Autodesk Inventor part; units mm, degrees
ref_plane "YZ Plane" through (0, 0, 0) normal (1, 0, 0) x (0, 1, 0)
ref_plane "XZ Plane" through (0, 0, 0) normal (0, 1, 0) x (-1, 0, 0)
ref_plane "XY Plane" through (0, 0, 0) normal (0, 0, 1) x (1, 0, 0)
sketch "Sketch1" plane through (0, 0, 0) normal (0, 0, 1) x (1, 0, 0)
  line L0 (0, -91.8925) -> (0, 152.1979) construction
  line L1 (3.18, 0) -> (7.58, 0)
  line L2 (7.58, 0) -> (7.58, 20)
  line L3 (7.58, 20) -> (3.18, 20)
  line L4 (3.18, 0) -> (3.18, 20)
  point P0 (0, 0)
  dimension "d1" = 3.18
  dimension "d2" = 20
  dimension "d17" = 4.4
  dimension "d18" = 7.58
revolve "Revolution1" add sketch "Sketch1" angle 360 about axis through (0, -91.8925, 0) along (0, 1, 0)
sketch "Sketch2" plane through (0, 0, 0) normal (0, 0, 1) x (1, 0, 0)
  line L0 (3.18, 0) -> (3.18, 20)
  line L1 (-7.58, 20) -> (7.58, 20) construction
  line L2 (7.58, 20) -> (42.58, 20) construction
  line L3 (7.58, 20) -> (7.58, 0)
  line L4 (38.7358, 38.6122) -> (39.7358, 38.6122)
  line L5 (38.7358, 38.6122) -> (33.7358, 38.6122)
  line L6 (39.7358, 38.6122) -> (39.7358, 43.6122)
  line L7 (33.7358, 38.6122) -> (33.7358, 43.6122)
  line L8 (39.7358, 43.6122) -> (41.7358, 43.6122)
  line L9 (41.7358, 43.6122) -> (41.7358, 36.6122)
  line L10 (41.7358, 36.6122) -> (7.58, 11.215)
  line L11 (33.7358, 43.6122) -> (31.7358, 43.6122)
  line L12 (3.18, 20) -> (7.58, 20)
  line L13 (7.58, 11.215) -> (7.58, 20)
  line L14 (0, 30.8602) -> (0, -63.1044)
  line L15 (31.7358, 43.6122) -> (31.7358, 40.4576)
  line L16 (31.7358, 40.4576) -> (3.18, 20)
  point P0 (0, 0)
  dimension "d6" = 35
  dimension "d7" = 1
  dimension "d8" = 5
  dimension "d9" = 5
  dimension "d10" = 5
  dimension "d11" = 2
  dimension "d12" = 7
  dimension "d13" = 2
revolve "Revolution2" add sketch "Sketch2" angle 360 about axis through (0, 30.8602, 0) along (0, -1, 0)
fillet "Fillet1" radius 2 1 edges at (-3.18, 20, 0)
fillet "Fillet2" radius 0.5 4 edges at (-31.7358, 43.6122, 0) (-33.7358, 43.6122, 0) (-39.7358, 43.6122, 0) (-41.7358, 43.6122, 0)
properties part number "Drain Funnel v0.6.2"
Part model, mm, in its own coordinate system. A direction names the side the tool comes from. Coordinates: 2 decimals unless noted, no trailing zeros. Order: outer loops, then holes, each group sorted by start corner. A loop starts at its lowest first (then second) coordinate and runs counter-clockwise, first axis right, second up. Notation, with made-up numbers: (-1.5, 57.25) -> (5.5, 57.25) arc R24 cw to (5.5, 73.25) -> close; hole circle Ø9 at (33.25, 55). An arc over 180 degrees is marked (long way). Put each result on its own line as item: value. Start each with the question number.
(1) Probe line 1 along Z through (x, y) = (0, 42); line 2 along X through (y, z) = (39.5, 14); line 3 along X through (y, z) = (41, 28). List the from-to ranges inside material, lowest first. Write a range as [from, to].
(2) Which spindle directions (+Z, -Z, +X, -X, +Y, -Y) get a long thin tool onto all of the face, cutting with end or side? Do faces 1 (the face through (7.23, 5.69, -2.28)), 2 (the face through (-33.12, 39.817, -25.396)), 3 (the face through (-26.77, 40.89, 20.53)). Say none if no direction does.
(3) Mould opens along X. For faces 4 (the face through (-18, 38.612, -29)), 5 (the face through (-5, 43.612, 32)), 6 (the face through (9.268, 12.804, -2.919)) say: pulls with the +X half, pulls with the -X half, needs draft (parallel to the pull), parting line crosses it, or undercut.
(4) Band-saw the part on A-A (y = 10). Give the cut face in (x, z), then the cut area to 3 significant figures.
(5) Pin check, flat tips, straight feed: pin 1 Ø8 at (x, y) = (12.5, 25.5) entering from +Z; pin 2 Ø4 at (x, z) = (29, 3) entering from -Y; pin 3 Ø2 at (x, z) = (-33, -14.5) entering from -Y; pin 4 Ø5.5 at (x, z) = (0, 0) entering from -Y (3 decimals). Stop position of each tip, or through.
(6) Band-saw the part on B-B (y = 34.5). Give the cut face in (x, z).
Determined:
1. line 1: z = [-41.74, -39.74], [-33.74, -31.74], [31.74, 33.74], [39.74, 41.74]
1. line 2: x = [-39.32, -37.19], [-30.69, -26.98], [26.98, 30.69], [37.19, 39.32]
1. line 3: x = [-30.95, -28.19], [-18.82, -14.94], [14.94, 18.82], [28.19, 30.95]
2. face 1: -Y
2. face 2: +Y, -Y
2. face 3: +Y
3. face 4: undercut
3. face 5: needs draft
3. face 6: parting line crosses it
4. outline: circle Ø15.16 at (0, 0); hole circle Ø6.36 at (0, 0)
4. area: 149 mm²
5. pin 1: stops at z = 29.86
5. pin 2: stops at y = 25.77
5. pin 3: stops at y = 31.64
5. pin 4: passes through
6. outline: circle Ø77.79 at (0, 0); hole circle Ø46.84 at (0, 0)
